from build123d import *

# Parameters (mm, degrees)
BOSS_EXTRUDE1_DEPTH     = 1.5875
SKETCH3_R               = 3.81
CUT_EXTRUDE1_DEPTH      = 2.5875
CUT_EXTRUDE1_DEPTH_BACK = 2.5875


with BuildPart() as part:
    # Sketch2 → Boss-Extrude1 (new body, symmetric)
    with BuildSketch(Plane(origin=(0, 0, 0), x_dir=(1, 0, 0), z_dir=(0, 1, 0))):
        Polygon((-596.116107134, 383.646334781), (0, 535.844392641), (596.116107134, 383.646334781), (853.792184287, 0), (596.116107134, -383.646334781), (0, -535.844392641), (-596.116107134, -383.646334781), (-853.792184287, 0), align=None)
        Polygon((-762, 0), (-549.079439398, 317.011162143), (0, 457.2), (549.079439398, 317.011162143), (762, 0), (549.079439398, -317.011162143), (0, -457.2), (-549.079439398, -317.011162143), align=None, mode=Mode.SUBTRACT)
    extrude(amount=BOSS_EXTRUDE1_DEPTH, both=True)

    # Sketch3 → Cut-Extrude1 (cut, two sides)
    with BuildSketch(Plane(origin=(0, 0, 0), x_dir=(1, 0, 0), z_dir=(0, 1, 0))) as cut_extrude1_sk:
        with Locations((690.246932705, 175.164374231)):
            Circle(SKETCH3_R)
        with Locations((690.246932705, -175.164374231)):
            Circle(SKETCH3_R)
        with Locations((-690.246932705, -175.164374231)):
            Circle(SKETCH3_R)
        with Locations((-690.246932705, 175.164374231)):
            Circle(SKETCH3_R)
        with Locations((-286.298886633, 423.425472391)):
            Circle(SKETCH3_R)
        with Locations((286.298886633, 423.425472391)):
            Circle(SKETCH3_R)
        with Locations((286.298886633, -423.425472391)):
            Circle(SKETCH3_R)
        with Locations((-286.298886633, -423.425472391)):
            Circle(SKETCH3_R)
    extrude(amount=CUT_EXTRUDE1_DEPTH, mode=Mode.SUBTRACT)
    extrude(cut_extrude1_sk.sketch, amount=-CUT_EXTRUDE1_DEPTH_BACK, mode=Mode.SUBTRACT)


solid = part.part
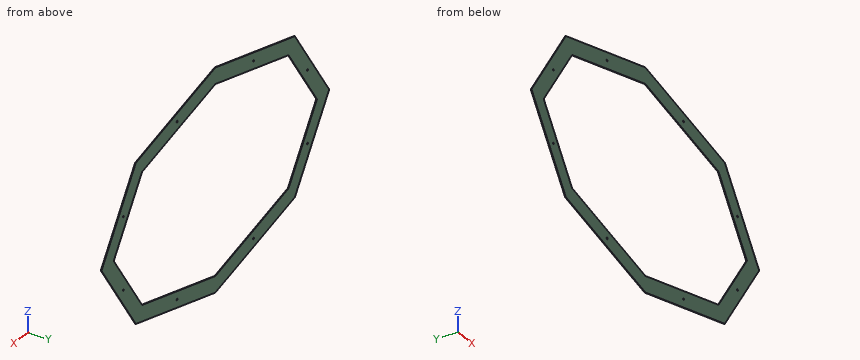
Geometry check sheet. Reference: the model listing, model coordinates, mm. Round coordinates to 2 decimals unless told otherwise and drop trailing zeros. Loops run counter-clockwise (first coordinate to the right, second up) from the corner with the lowest first, then second, coordinate; pieces in that order, holes last. Notation, with made-up numbers: (18, 55) - (36, 55) arc R21 ccw to (36, 85) - close; hole circle Ø4 at (83, 73.25). An arc over 180 degrees is marked (long way). Answer as CSV lines item,"result".
(1) Material ranges on line 1 along Z through (x, y) = (690.5, -1.25); line 2 along Z through (x, y) = (657, 0.4); line 3 along Z through (x, y) = (-223.5, -1.25), recorded low to high.
Output values:
line 1,"z = -243.12 to -178.97, -171.36 to -106.45, 106.45 to 171.36, 178.97 to 243.12"
line 2,"z = -293 to -156.33, 156.33 to 293"
line 3,"z = -478.78 to -400.14, 400.14 to 478.78"
(2) Cross-section at B-B, the plane z = 253. Enter the section's corners in (x, y), and give its area (3 significant figures).
Output values:
outline,"(-683.86, -1.59) - (-592.07, -1.59) - (-592.07, 1.59) - (-683.86, 1.59) - close; (592.07, -1.59) - (683.86, -1.59) - (683.86, 1.59) - (592.07, 1.59) - close"
area,"583 mm²"
(3) Depth check by flat-ended pin: pin 1 Ø4.5 at (x, z) = (-286.3, -423.43) entering from -Y; pin 2 Ø1 at (x, y) = (103.5, 0.5) entering from -Z. Enter the tip coordinate at first touch or a pass-through.
Output values:
pin 1,"passes through"
pin 2,"stops at z = -509.55"
(4) Cross-section at C-C, the plane y = 0.7. Give the number of separate pieces and of enclosed holes in the cut face, and give its area (3 significant figures).
Output values:
separate pieces,"1"
enclosed holes,"9"
area,"308,000 mm²"
(5) Cross-section at A-A, the plane x = 613.5. Enter the section's corners in (y, z).
Output values:
outline,"(-1.59, -357.76) - (1.59, -357.76) - (1.59, -221.1) - (-1.59, -221.1) - close; (-1.59, 221.1) - (1.59, 221.1) - (1.59, 357.76) - (-1.59, 357.76) - close"
